Source: CAD feature listing. Evaluate the final solid. Frame: model axes, mm. Give positions to 0.01 mm unless a question says otherwise; leave off trailing zeros. Order: outer loops, then holes, each group sorted by start corner. A loop starts at its lowest first (then second) coordinate and runs counter-clockwise, first axis right, second up.
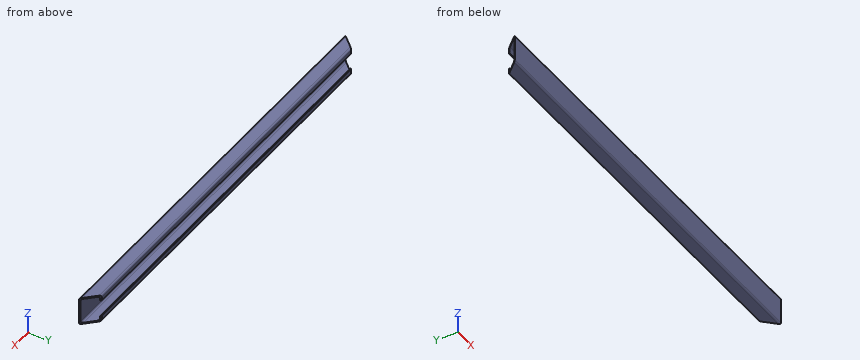
from build123d import *

# Parameters (mm, degrees)
RESSALTO_EXTRUS_O1_DEPTH = 1500
FILETE1_R                = 6
CORTE_EXTRUS_O1_DEPTH    = 50
CORTE_EXTRUS_O2_DEPTH    = 50


with BuildPart() as part:
    # Esboço1 → Ressalto-extrusão1 (new body)
    with BuildSketch(Plane(origin=(0, 0, 0), x_dir=(0, 0, -1), z_dir=(1, 0, 0))):
        Polygon((-46, 21), (-46, -21), (46, -21), (46, 21), (30, 21), (30, 25), (50, 25), (50, -25), (-50, -25), (-50, 25), (-30, 25), (-30, 21), align=None)
    extrude(amount=RESSALTO_EXTRUS_O1_DEPTH)

    # Filete1
    filete1_edges = [part.edges().sort_by_distance(p)[0] for p in [
        (750, -25, -50),
        (750, -25, 50),
        (750, 25, 50),
        (750, 21, 46),
        (750, -21, 46),
        (750, -21, -46),
        (750, 21, -46),
        (750, 25, -50),
    ]]
    fillet(filete1_edges, radius=FILETE1_R)

    # Esboço3 → Corte-extrusão1 (cut, symmetric)
    with BuildSketch(Plane.XY):
        Polygon((0, -25), (184.767559257, 159.767559257), (-208.615442636, 104.939092506), align=None)
        Polygon((1500, -25), (1327.707280818, 147.292719182), (1799.383443157, 147.292719182), align=None)
    extrude(amount=CORTE_EXTRUS_O1_DEPTH, both=True, mode=Mode.SUBTRACT)

    # Esboço4 → Corte-extrusão2 (cut, symmetric)
    with BuildSketch(Plane.XY):
        Polygon((50, 25), (-16.235639867, -48.562130564), (-42.129730134, -17.715767118), align=None)
    extrude(amount=CORTE_EXTRUS_O2_DEPTH, both=True, mode=Mode.SUBTRACT)


solid = part.part
1) Section query C-C on z = 5.5. Output: boundary loops of the cut face in (x, y).
Checks:
outline: (4.98, -25) - (1500, -25) - (1496, -21) - (8.58, -21) - close
2) Section query B-B on x = 462.5. Output: boundary loops of the cut face in (y, z).
Checks:
outline: (-25, -44) arc R6 ccw to (-19, -50) - (19, -50) arc R6 ccw to (25, -44) - (25, -30) - (21, -30) - (21, -40) arc R6 cw to (15, -46) - (-15, -46) arc R6 cw to (-21, -40) - (-21, 40) arc R6 cw to (-15, 46) - (15, 46) arc R6 cw to (21, 40) - (21, 30) - (25, 30) - (25, 44) arc R6 ccw to (19, 50) - (-19, 50) arc R6 ccw to (-25, 44) - close
3) Section query A-A on y = 3.5. Output: boundary loops of the cut face in (x, z), and give its area (3 significant figures).
Checks:
outline: (30.64, -50) - (1471.5, -50) - (1471.5, -46) - (30.64, -46) - close; (30.64, 46) - (1471.5, 46) - (1471.5, 50) - (30.64, 50) - close
area: 11,500 mm2
4) Ray query, L1, parallel to Z at x = 882.5, y = 7; L2, parallel to Z at x = 461, y = 16.5; L3, parallel to Y at x = 246, z = 33. Return the intervals inside material, ascending.
Checks:
L1: z = -50 to -46, 46 to 50
L2: z = -50 to -45.81, 45.81 to 50
L3: y = -25 to -21, 21 to 25
5) First-contact query: pin 1 Ø4 at (x, z) = (1210, 13) entering from +Y; pin 2 Ø1.2 at (x, y) = (918, 22) entering from +Z; pin 3 Ø4.5 at (x, y) = (980, 22.5) entering from -Z. Flat tips, straight axial feed; report the tip coordinate or a pass-through.
Checks:
pin 1: stops at y = -21
pin 2: stops at z = 49.5
pin 3: stops at z = -49.87
